from build123d import *

# Parameters (mm, degrees)
SKETCH2_R           = 1.7
SKETCH2_R_2         = 5
BOSS_EXTRUDE4_DEPTH = 3


with BuildPart() as part:
    # Sketch2 → Boss-Extrude4 (new body)
    with BuildSketch(Plane.XY):
        with BuildLine():
            Line((-49.411099801, -41.712890537), (-34.411099801, -26.724072871))
            Line((-34.411099801, -26.724072871), (56.012900199, -26.724072871))
            Line((56.012900199, -26.724072871), (71.012900199, -41.724072871))
            Line((71.012900199, -41.724072871), (95.012900199, -41.724072871))
            ThreePointArc((95.012900199, -41.724072871), (102.06743807, -44.301892558), (105.013826091, -51.210615779))
            Line((105.013826091, -51.210615779), (105.009259778, -101.753736116))
            ThreePointArc((105.009259778, -101.753736116), (102.047198601, -108.629676096), (95.012900199, -111.193072871))
            Line((95.012900199, -111.193072871), (71.012900199, -111.193072871))
            Line((71.012900199, -111.193072871), (56.012900199, -126.193072871))
            Line((56.012900199, -126.193072871), (-34.411099801, -126.193072871))
            Line((-34.411099801, -126.193072871), (-49.411099801, -111.193072871))
            Line((-49.411099801, -111.193072871), (-73.411099801, -111.193072871))
            ThreePointArc((-73.411099801, -111.193072871), (-80.170723963, -108.333415965), (-83.411099801, -101.747816457))
            Line((-83.411099801, -101.747816457), (-83.411099801, -51.162112892))
            ThreePointArc((-83.411099801, -51.162112892), (-80.443251923, -44.29297937), (-73.411099801, -41.735255206))
            Line((-73.411099801, -41.735255206), (-49.411099801, -41.712890537))
        make_face()
        with Locations((-49.411099801, -61.458572871)):
            Circle(SKETCH2_R, mode=Mode.SUBTRACT)
        with Locations((-73.411099801, -61.458572871)):
            Circle(SKETCH2_R, mode=Mode.SUBTRACT)
        with Locations((-73.411099801, -91.458572871)):
            Circle(SKETCH2_R, mode=Mode.SUBTRACT)
        with Locations((-49.411099801, -91.458572871)):
            Circle(SKETCH2_R, mode=Mode.SUBTRACT)
        with Locations((95.012900199, -91.458572871)):
            Circle(SKETCH2_R, mode=Mode.SUBTRACT)
        with Locations((71.012900199, -91.458572871)):
            Circle(SKETCH2_R, mode=Mode.SUBTRACT)
        with Locations((95.012900199, -61.458572871)):
            Circle(SKETCH2_R, mode=Mode.SUBTRACT)
        with Locations((71.012900199, -61.458572871)):
            Circle(SKETCH2_R, mode=Mode.SUBTRACT)
        with Locations((10.800900199, -76.383042082)):
            Circle(SKETCH2_R_2, mode=Mode.SUBTRACT)
        with Locations((-34.411099801, -41.724072871)):
            Circle(SKETCH2_R, mode=Mode.SUBTRACT)
        with Locations((-34.411099801, -111.193072871)):
            Circle(SKETCH2_R, mode=Mode.SUBTRACT)
        with Locations((56.012900199, -111.193072871)):
            Circle(SKETCH2_R, mode=Mode.SUBTRACT)
        with Locations((56.012900199, -41.724072871)):
            Circle(SKETCH2_R, mode=Mode.SUBTRACT)
    extrude(amount=BOSS_EXTRUDE4_DEPTH)


solid = part.part
Geometry check sheet. Reference: the model listing, model coordinates, mm. Coordinates: 2 decimals unless noted, no trailing zeros. Order: outer loops, then holes, each group sorted by start corner. A loop starts at its lowest first (then second) coordinate and runs counter-clockwise, first axis right, second up. Notation, with made-up numbers: (32.25, -10.75) -> (79.25, -10.75) arc R14 cw to (79.25, -0.75) -> close; hole circle Ø6 at (53, 46.5). An arc over 180 degrees is marked (long way). Use a Markdown table: item, result. Add a question column.
1. Material ranges on L1, parallel to X at y = -91.5, z = 2.8; L2, parallel to Y at x = 69.5, z = 2.55; L3, parallel to Y at x = 55, z = 1.65, recorded low to high.
2. Cross-section at C-C (y = -119.5). Enter the section's corners in (x, z), and give its area (3 significant figures).
3. Go/stop test with flat-tipped pins: pin 1 Ø1.5 at (y, z) = (-86, 1) entering from +X; pin 2 Ø0.9 at (x, z) = (88.5, 2) entering from +Y. Record where each tip stops, or that it passes through.
4. Mould release check, pull along X, two halves, no side actions. Record for faces 1 (the face through (12, -65, 0)), 2 (the face through (-34.632, -109.508, 1.479)), 3 (the face through (-42.016, -34.323, 1.479)), 4 (the face through (-35.664, -40.575, 1.479)): pulls with the +X half, pulls with the -X half, needs draft (parallel to the pull), parting line crosses it, or undercut.
5. Cross-section at A-A (z = 2.4). Give the number of separate pieces and of enclosed holes in the cut face, and give its area (3 significant figures).
6. Cross-section at B-B (x = 81). Enter the section's corners in (y, z).
Filled sheet:
| question | item | result |
|---|---|---|
| 1 | L1 | -83.41 to -75.11, -71.71 to -51.11, -47.71 to 69.31, 72.71 to 93.31, 96.71 to 105.01 |
| 1 | L2 | -112.71 to -92.23, -90.68 to -62.23, -60.68 to -40.21 |
| 1 | L3 | -126.19 to -112.56, -109.83 to -43.09, -40.36 to -26.72 |
| 2 | outline | (-41.1, 0) -> (62.71, 0) -> (62.71, 3) -> (-41.1, 3) -> close |
| 2 | area | 311 mm2 |
| 3 | pin 1 | x = 105.01 |
| 3 | pin 2 | y = -41.72 |
| 4 | face 1 | needs draft |
| 4 | face 2 | undercut |
| 4 | face 3 | pulls with the -X half |
| 4 | face 4 | undercut |
| 5 | separate pieces | 1 |
| 5 | enclosed holes | 13 |
| 5 | area | 16,000 mm2 |
| 6 | outline | (-111.19, 0) -> (-41.72, 0) -> (-41.72, 3) -> (-111.19, 3) -> close |
